Geometry: final body of the model. Coordinates: model frame, mm. Face numbers are marked on the shaded views. A direction names the side the tool comes from. Give positions to 0.01 mm unless a question says otherwise; leave off trailing zeros. Write each loop counter-clockwise with the first axis right and the second up, starting at its lowest first coordinate (ties: lowest second). Pieces come first, ordered by that corner, then holes. Notation, with made-up numbers: M -3,35.5 L 44,35.5 A22 cw 44,69.5 Z; hole C 57.25,-12 d4. An arc over 180 degrees is marked long. Use a Markdown table: item, result. Add a question column.
1) Pin query (flat end, axial travel): pin 1 (4 mm diameter, centred on y = 30.5, z = -87.5, fed in from +X); pin 2 (10 mm diameter, centred on y = 30.5, z = -10.5, fed in from -X); pin 3 (4 mm diameter, centred on x = -104, y = 30.5, fed in from +Z). Return the tip coordinate at first contact, or that it passes through.
2) Set-up query: the marked faces 1 and 2. Return all of +Z, -Z, +X, -X, +Y, -Y with unobstructed straight access to the full face (end or side cutting, diameter ignored); none if empty.
3) Section A-A on y = 30. Return the cut outline in (x, z), then the cut area to 3 significant figures.
4) Line query: line 1 (Z direction, x = -19, y = 35); line 2 (Y direction, x = -12.7, z = -58); line 3 (X direction, y = 6.35, z = -52). Output: solid intervals per line, ascending.
5) Section B-B on z = -41. Return the cut outline in (x, y).
6) Draft query along Z for the marked faces 3, 4 and 5. Return one class per face: +Z half, -Z half, draft (parallel to the pull), parting line (faces both ways), or undercut.
7) Section C-C on x = -101. Return the cut outline in (y, z), then the cut area to 3 significant figures.
8) Section D-D on z = -88. Return the cut outline in (x, y), then the cut area to 3 significant figures.
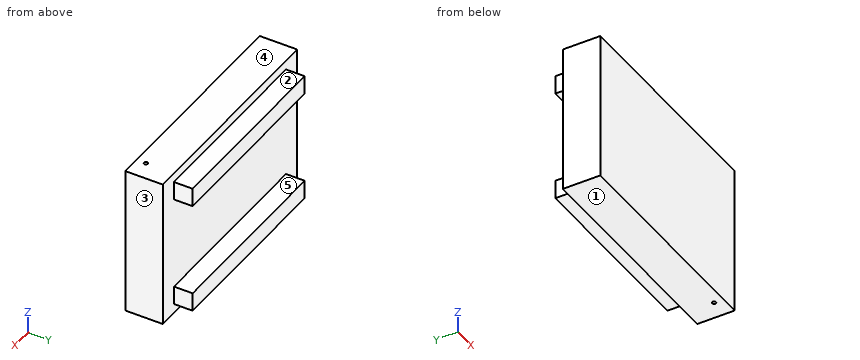
Autodesk Inventor part; units mm, degrees
ref_plane "Work Plane1" through (-152.4, 0, -50.8) normal (0, 0, 1) x (1, 0, 0)
ref_plane "YZ Plane" through (0, 0, 0) normal (1, 0, 0) x (0, 1, 0)
ref_plane "XZ Plane" through (0, 0, 0) normal (0, 1, 0) x (-1, 0, 0)
sketch "Sketch1" plane through (0, 0, 0) normal (0, 1, 0) x (-1, 0, 0)
  line L0 (0, 0) -> (152.4, 0)
  line L1 (152.4, 0) -> (152.4, -101.6)
  line L2 (152.4, -101.6) -> (0, -101.6)
  line L3 (0, -101.6) -> (0, 0)
  dimension "d0" = 152.4
  dimension "d1" = 101.6
extrude "Extrusion1" add sketch "Sketch1" along normal blind 38.1
ref_plane "Work Plane1" through (-152.4, 0, -50.8) normal (0, 0, 1) x (1, 0, 0)
sketch "Sketch3" plane through (0, 38.1, 0) normal (0, 1, 0) x (1, 0, 0)
  line L0 (-139.7, 95.25) -> (-12.7, 95.25)
  line L1 (-12.7, 95.25) -> (-12.7, 82.55)
  line L2 (-12.7, 82.55) -> (-139.7, 82.55)
  line L3 (-139.7, 82.55) -> (-139.7, 95.25)
  line L4 (0, 101.6) -> (-152.4, 101.6)
  line L5 (0, 0) -> (0, 101.6)
  line L6 (-152.4, 101.6) -> (-152.4, 0)
  line L7 (30.48, 50.8) -> (-182.88, 50.8)
  line L8 (-139.7, 6.35) -> (-12.7, 6.35)
  line L9 (-12.7, 6.35) -> (-12.7, 19.05)
  line L10 (-12.7, 19.05) -> (-139.7, 19.05)
  line L11 (-139.7, 19.05) -> (-139.7, 6.35)
  line L12 (0, 101.6) -> (-152.4, 101.6)
  line L13 (-152.4, 101.6) -> (-152.4, 0)
  line L14 (-152.4, 0) -> (0, 0)
  line L15 (0, 0) -> (0, 101.6)
  dimension "d12" = 6.35
  dimension "d13" = 12.7
  dimension "d14" = 12.7
  dimension "d15" = 12.7
extrude "Extrusion3" cut sketch "Sketch3" against normal blind 12.7
sketch "Sketch4" plane through (0, 0, -101.6) normal (0, 0, -1) x (-1, 0, 0)
  line L0 (0, 0) -> (0, 25.4)
  line L1 (152.4, 0) -> (0, 0)
  point P0 (12.7, 6.35)
  dimension "d18" = 12.7
  dimension "d19" = 6.35
hole "Hole1" at (-12.7, 6.35, -101.6) direction (0, 0, 1) diameter 2.54 end through all
properties part number "BS #3"
Found:
| question | item | result |
|---|---|---|
| 1 | pin 1 | x = -12.7 |
| 1 | pin 2 | x = -139.7 |
| 1 | pin 3 | z = -6.35 |
| 2 | face 1 | -Z, +X, -X, +Y, -Y |
| 2 | face 2 | +Z, +X, -X, +Y |
| 3 | outline | M -139.7,-95.25 L -12.7,-95.25 L -12.7,-82.55 L -139.7,-82.55 Z; M -139.7,-19.05 L -12.7,-19.05 L -12.7,-6.35 L -139.7,-6.35 Z |
| 3 | area | 3,230 mm² |
| 4 | line 1 | -95.25 to -82.55, -19.05 to -6.35 |
| 4 | line 2 | 0 to 5.08, 7.62 to 25.4 |
| 4 | line 3 | -152.4 to -13.97, -11.43 to 0 |
| 5 | outline | M -152.4,0 L 0,0 L 0,25.4 L -152.4,25.4 Z; hole C -12.7,6.35 d2.54 |
| 6 | face 3 | draft |
| 6 | face 4 | +Z half |
| 6 | face 5 | undercut |
| 7 | outline | M 0,-101.6 L 25.4,-101.6 L 25.4,-95.25 L 38.1,-95.25 L 38.1,-82.55 L 25.4,-82.55 L 25.4,-19.05 L 38.1,-19.05 L 38.1,-6.35 L 25.4,-6.35 L 25.4,0 L 0,0 Z |
| 7 | area | 2,900 mm² |
| 8 | outline | M -152.4,0 L 0,0 L 0,25.4 L -12.7,25.4 L -12.7,38.1 L -139.7,38.1 L -139.7,25.4 L -152.4,25.4 Z; hole C -12.7,6.35 d2.54 |
| 8 | area | 5,480 mm² |
